Model file for the job. Use its own axes, mm. Face numbers are marked on the shaded views. A direction names the side the tool comes from. Round coordinates to 2 decimals unless told otherwise and drop trailing zeros. Order: outer loops, then holes, each group sorted by start corner. A loop starts at its lowest first (then second) coordinate and runs counter-clockwise, first axis right, second up. Notation, with made-up numbers: (2, -18.5) - (24, -18.5) arc R24 cw to (24, -1.5) - close; hole circle Ø3 at (38, 6). An arc over 180 degrees is marked (long way). Put each result on its own line as item: value. Start each with the question number.
Item 1: Pin check, flat tips, straight feed: pin 1 Ø5 at (x, y) = (68, 11.5) entering from -Z; pin 2 Ø1.5 at (x, y) = (65, -8) entering from +Z; pin 3 Ø8 at (x, y) = (18.5, 10) entering from +Z. Stop position of each tip, or through.
Item 2: Saw through at A-A on z = 0. List the corners of the cut face in (x, y), plus the area to 3 significant figures.
Item 3: Saw through at C-C on x = 9. List the corners of the cut face in (y, z), plus the area to 3 significant figures.
Item 4: Which spindle directions (+Z, -Z, +X, -X, +Y, -Y) get a long thin tool onto all of the face, cutting with end or side? Do the marked faces 1 and 2. Say none if no direction does.
Item 5: Mould opens along Y. For the marked faces 3 and 4 say: pulls with the +Y half, pulls with the -Y half, needs draft (parallel to the pull), parting line crosses it, or undercut.
Item 6: Probe probe 1 along X at (y, z) = (3.25, -13.5); probe 2 along Z at (x, y) = (67, -8); probe 3 along Z at (x, y) = (11, 3.5). List the from-to ranges inside material, lowest first.
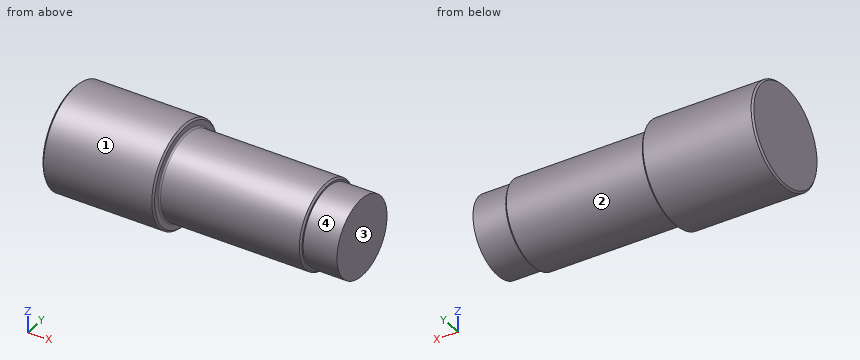
```python
from build123d import *

# Parameters (mm, degrees)
SKETCH_1_R      = 15
EXTRUDE_1_DEPTH = 33
SKETCH_2_R      = 12.5
EXTRUDE_2_DEPTH = 42
FILLET_1_R      = 0.5
CHAMFER_1_SIZE  = 0.5
SKETCH_3_R      = 11.5
EXTRUDE_3_DEPTH = 10


with BuildPart() as part:
    # 草图1 → 凸台-拉伸1 (new body)
    with BuildSketch(Plane(origin=(0, 0, 0), x_dir=(0, 0, -1), z_dir=(1, 0, 0))):
        Circle(SKETCH_1_R)
    extrude(amount=EXTRUDE_1_DEPTH)

    # 草图2 → 凸台-拉伸2 (add)
    with BuildSketch(Plane(origin=(33, 0, 0), x_dir=(0, 0, -1), z_dir=(1, 0, 0))):
        Circle(SKETCH_2_R)
    extrude(amount=EXTRUDE_2_DEPTH)

    # 圆角1
    fillet_1_edges = [part.edges().sort_by_distance(p)[0] for p in [
        (33, 0, 12.5),
    ]]
    fillet(fillet_1_edges, radius=FILLET_1_R)

    # 倒角1
    chamfer_1_edges = [part.edges().sort_by_distance(p)[0] for p in [
        (0, 0, 15),
        (33, 0, 15),
        (75, 0, 12.5),
    ]]
    chamfer(chamfer_1_edges, length=CHAMFER_1_SIZE)

    # 草图3 → 凸台-拉伸3 (add)
    with BuildSketch(Plane(origin=(75, 0, 0), x_dir=(0, 0, -1), z_dir=(1, 0, 0))):
        Circle(SKETCH_3_R)
    extrude(amount=EXTRUDE_3_DEPTH)


solid = part.part
```
Results found:
1. pin 1: stops at z = -8.67
1. pin 2: stops at z = 10.18
1. pin 3: stops at z = 13.75
2. outline: (0, -14.5) - (0.5, -15) - (32.5, -15) - (33, -14.5) - (33, -13) arc R0.5 cw to (33.5, -12.5) - (74.5, -12.5) - (75, -12) - (75, -11.5) - (85, -11.5) - (85, 11.5) - (75, 11.5) - (75, 12) - (74.5, 12.5) - (33.5, 12.5) arc R0.5 cw to (33, 13) - (33, 14.5) - (32.5, 15) - (0.5, 15) - (0, 14.5) - close
2. area: 2,270 mm²
3. outline: circle Ø30 at (0, 0)
3. area: 707 mm²
4. face 1: +X, -X
4. face 2: +X
5. face 3: needs draft
5. face 4: parting line crosses it
6. probe 1: x = 0 to 33
6. probe 2: z = -9.6 to 9.6
6. probe 3: z = -14.59 to 14.59
